from build123d import *

# Parameters (mm, degrees)
SKETCH_W     = 17
SKETCH_H     = 56
SKETCH_R     = 2.5
PAD_DEPTH    = 3
SKETCH001_W  = 3
SKETCH001_H  = 16
PAD001_DEPTH = 5
FILLET_R     = 3


with BuildPart() as part:
    # Sketch → Pad (new body)
    with BuildSketch(Plane.XY):
        with Locations((8.5, 8)):
            Rectangle(SKETCH_W, SKETCH_H)
        with Locations((7, 28)):
            Circle(SKETCH_R, mode=Mode.SUBTRACT)
        with Locations((7, -12)):
            Circle(SKETCH_R, mode=Mode.SUBTRACT)
    extrude(amount=PAD_DEPTH)

    # Sketch001 → Pad001 (join)
    with BuildSketch(Plane.XY):
        with Locations((15.5, 8)):
            Rectangle(SKETCH001_W, SKETCH001_H)
    extrude(amount=PAD001_DEPTH)

    # Fillet
    fillet_edges = [part.edges().sort_by_distance(p)[0] for p in [
        (17, -20, 1.5),
        (0, -20, 1.5),
        (17, 36, 1.5),
        (0, 36, 1.5),
    ]]
    fillet(fillet_edges, radius=FILLET_R)


solid = part.part
Build history of the part. All positions in model axes, mm. A direction names the side the tool comes from. Round coordinates to 2 decimals unless told otherwise and drop trailing zeros. Loops run counter-clockwise (first coordinate to the right, second up) from the corner with the lowest first, then second, coordinate; pieces in that order, holes last. Notation, with made-up numbers: (85.25, 36) -> (96.25, 36) arc R18 cw to (96.25, 60) -> close; hole circle Ø1 at (55.25, -8). An arc over 180 degrees is marked (long way). Answer in a Markdown table with one row per item.
Item 1: Mould opens along X. For faces 1 (the cylindrical face through (0.86, 35.1, 1.52)), 2 (the cylindrical face through (8.15, -14.22, 1.48)), 3 (the cylindrical face through (16.1, 35.14, 1.52)) say: +X half, -X half, draft (parallel to the pull), parting line (faces both ways), or undercut.
Answers below:
| item | result |
|---|---|
| face 1 | -X half |
| face 2 | undercut |
| face 3 | +X half |
Item 2: Drill centre lines: L1, parallel to Y at x = 7, z = 2.25; L2, parallel to Z at x = 1.25, y = -1; L3, parallel to X at y = 1, z = 4.6. Where is each one in solid material? Low to high. Write a range as [from, to].
Answers below:
| item | result |
|---|---|
| L1 | y = [-20, -14.5], [-9.5, 25.5], [30.5, 36] |
| L2 | z = [0, 3] |
| L3 | x = [14, 17] |
Item 3: Saw through at D-D (x = 15). Write the cut outline in (y, z), and give its area (3 significant figures).
Answers below:
| item | result |
|---|---|
| outline | (-19.83, 0) -> (35.83, 0) -> (35.83, 3) -> (16, 3) -> (16, 5) -> (0, 5) -> (0, 3) -> (-19.83, 3) -> close |
| area | 199 mm² |
Item 4: Saw through at C-C (z = 0.8). Write the cut outline in (x, y).
Answers below:
| item | result |
|---|---|
| outline | (0, -17) arc R3 ccw to (3, -20) -> (14, -20) arc R3 ccw to (17, -17) -> (17, 33) arc R3 ccw to (14, 36) -> (3, 36) arc R3 ccw to (0, 33) -> close; hole circle Ø5 at (7, -12); hole circle Ø5 at (7, 28) |
Item 5: Saw through at B-B (y = -12). Write the cut outline in (x, z), and give its area (3 significant figures).
Answers below:
| item | result |
|---|---|
| outline | (0, 0) -> (4.5, 0) -> (4.5, 3) -> (0, 3) -> close; (9.5, 0) -> (17, 0) -> (17, 3) -> (9.5, 3) -> close |
| area | 36.0 mm² |
Item 6: Saw through at A-A (x = 7). Write the cut outline in (y, z).
Answers below:
| item | result |
|---|---|
| outline | (-20, 0) -> (-14.5, 0) -> (-14.5, 3) -> (-20, 3) -> close; (-9.5, 0) -> (25.5, 0) -> (25.5, 3) -> (-9.5, 3) -> close; (30.5, 0) -> (36, 0) -> (36, 3) -> (30.5, 3) -> close |
Item 7: Which spindle directions (+Z, -Z, +X, -X, +Y, -Y) get a long thin tool onto all of the face, cutting with end or side? Do faces 4 (the flat face through (14, 8, 4)), 5 (the flat face through (15, 16, 4)), 6 (the flat face through (15, 0, 4)). Say none if no direction does.
Answers below:
| item | result |
|---|---|
| face 4 | +Z, -X, +Y, -Y |
| face 5 | +Z, +X, -X, +Y |
| face 6 | +Z, +X, -X, -Y |
Item 8: Pin check, flat tips, straight feed: pin 1 (5 mm diameter, centred on x = 9, y = -5, fed in from +Z); pin 2 (1 mm diameter, centred on x = 16, z = 4, fed in from -Y); pin 3 (1.6 mm diameter, centred on y = 9.5, z = 4, fed in from -X); pin 4 (3 mm diameter, centred on x = 7, y = 28, fed in from +Z). Stop position of each tip, or through.
Answers below:
| item | result |
|---|---|
| pin 1 | stops at z = 3 |
| pin 2 | stops at y = 0 |
| pin 3 | stops at x = 14 |
| pin 4 | passes through |
